For this review, take the finished solid that the model builds, in its own axes (mm). A direction names the side the tool comes from. Coordinates: 2 decimals unless noted, no trailing zeros. Write each loop counter-clockwise with the first axis right and the second up, starting at its lowest first coordinate (ties: lowest second). Pieces come first, ordered by that corner, then holes. Notation, with made-up numbers: M 66,52.5 L 102,52.5 A33 cw 102,90.5 Z; hole C -7.75,-19 d3. An arc over 180 degrees is marked long. One line per question, with ' | ' between items.
from build123d import *

# Parameters (mm, degrees)
SKETCH_1_R          = 10
SKETCH_1_R_2        = 1.5
EXTRUDE_2_DEPTH     = 2
SKETCH_2_R          = 4.5
EXTRUDE_3_DEPTH     = 2.9
CHAMFER_1_SIZE      = 0.4
SKETCH_5_R          = 1.5
CUT_EXTRUDE_1_DEPTH = 10


with BuildPart() as part:
    # 草图1 → 凸台-拉伸2 (new body)
    with BuildSketch(Plane(origin=(0, 0, 0), x_dir=(1, 0, 0), z_dir=(0, 1, 0))):
        with Locations(Location((0, 0, 0), (0, 0, 270))):
            Circle(SKETCH_1_R)
        with Locations(Location((0, 7, 0), (0, 0, 270))):
            Circle(SKETCH_1_R_2, mode=Mode.SUBTRACT)
        with Locations(Location((7, 0, 0), (0, 0, 270))):
            Circle(SKETCH_1_R_2, mode=Mode.SUBTRACT)
        with Locations(Location((-7, 0, 0), (0, 0, 270))):
            Circle(SKETCH_1_R_2, mode=Mode.SUBTRACT)
        with Locations(Location((0, -7, 0), (0, 0, 270))):
            Circle(SKETCH_1_R_2, mode=Mode.SUBTRACT)
    extrude(amount=EXTRUDE_2_DEPTH)

    # 草图2 → 凸台-拉伸3 (add)
    with BuildSketch(Plane(origin=(0, 0, 0), x_dir=(1, 0, 0), z_dir=(0, 1, 0))):
        with Locations(Location((0, 0, 0), (0, 0, 270))):
            Circle(SKETCH_2_R)
        Polygon((2.5, 0), (2.976344104, 0.375999701), (2.421457903, 0.621724718), (2.789329458, 1.104373658), (2.1907667, 1.204384185), (2.427050983, 1.763355757), (1.822421569, 1.711367765), (1.912271969, 2.311539728), (1.339566987, 2.110819814), (1.277337875, 2.714481157), (0.772542486, 2.377641291), (0.562143944, 2.946861752), (0.156976299, 2.495066821), (-0.188371559, 2.994080185), (-0.468453286, 2.455718127), (-0.927050983, 2.853169549), (-1.064448229, 2.262067631), (-1.607480385, 2.532983777), (-1.593559974, 1.926283107), (-2.186905882, 2.053641318), (-2.022542486, 1.469463131), (-2.62892004, 1.445261022), (-2.324441215, 0.920311382), (-2.905749483, 0.746069661), (-2.480286753, 0.313333084), (-3, 0), (-2.480286753, -0.313333084), (-2.905749483, -0.746069661), (-2.324441215, -0.920311382), (-2.62892004, -1.445261022), (-2.022542486, -1.469463131), (-2.186905882, -2.053641318), (-1.593559974, -1.926283107), (-1.607480385, -2.532983777), (-1.064448229, -2.262067631), (-0.927050983, -2.853169549), (-0.468453286, -2.455718127), (-0.188371559, -2.994080185), (0.156976299, -2.495066821), (0.562143944, -2.946861752), (0.772542486, -2.377641291), (1.277337875, -2.714481157), (1.339566987, -2.110819814), (1.912271969, -2.311539728), (1.822421569, -1.711367765), (2.427050983, -1.763355757), (2.1907667, -1.204384185), (2.789329458, -1.104373658), (2.421457903, -0.621724718), (2.976344104, -0.375999701), align=None, mode=Mode.SUBTRACT)
    extrude(amount=-EXTRUDE_3_DEPTH)

    # 草图4 → 切除-旋转1 (revolve, cut)
    with BuildSketch(Plane.XY):
        Polygon((0, -2.9), (0, -2.128896783), (2.5, -2.128896783), (3.136710161, -2.9), align=None)
    revolve(axis=Axis((0, -2.9, 0), (0, 1, 0)), mode=Mode.SUBTRACT)

    # 倒角1
    chamfer_1_edges = [part.edges().sort_by_distance(p)[0] for p in [
        (0, 0, -10),
        (0, 2, -10),
    ]]
    chamfer(chamfer_1_edges, length=CHAMFER_1_SIZE)

    # 草图5 → 切除-拉伸1 (cut)
    with BuildSketch(Plane(origin=(0, 0, 0), x_dir=(1, 0, 0), z_dir=(0, 1, 0))):
        with Locations(Location((0, 0, 0), (0, 0, 270))):
            Circle(SKETCH_5_R)
    extrude(amount=CUT_EXTRUDE_1_DEPTH, mode=Mode.SUBTRACT)


solid = part.part
1. For line 1 along Z through (x, y) = (-0.25, 1); line 2 along Y through (x, z) = (-3.5, 6.5); line 3 along Z through (x, y) = (8, 1.15), list the stretches that pass through material, from the lowest coordinate up.
Computed values:
line 1: z = -10 to -8.48, -5.52 to -1.48, 1.48 to 5.52, 8.48 to 10 | line 2: y = 0 to 2 | line 3: z = -6 to -1.12, 1.12 to 6
2. Machinability: for faces 1 (the cylindrical face through (0.07, 0.99, -8.5)), 2 (the flat face through (2.3, 0, 4.1)), which of the approach directions +Z, -Z, +X, -X, +Y, -Y give a long, thin tool a straight path to every point of the face, cutting with its end or side? Answer none if there is none.
Computed values:
face 1: +Y, -Y | face 2: -Y
3. Take a section at A-A on y = 0.65. State the section outline as (x, z) points.
Computed values:
outline: C 0,0 d20; hole C -7,0 d3; hole C 0,-7 d3; hole C 0,0 d3; hole C 0,7 d3; hole C 7,0 d3
4. Clearance check with flat-ended pins moving along their axes: P1, Ø1.5, axis at x = 3, y = -2, coming from the -Z side; P2, Ø1, axis at x = 4.5, y = 1, coming from the -Z side. State where each tip first meets the part, or that it passes through.
Computed values:
P1: stops at z = -3.9 | P2: stops at z = -9.17
5. Draft analysis for pull direction X (two halves, no side actions). For faces 3 (the cylindrical face through (1.352, -1.43, 4.292)), 4 (the cylindrical face through (0.45, 0.99, 1.43)), 5 (the flat face through (0, 2, 2)), state which applies: pulls with the +X half, pulls with the -X half, needs draft (parallel to the pull), parting line crosses it, or undercut.
Computed values:
face 3: parting line crosses it | face 4: undercut | face 5: needs draft
